from build123d import *

# Parameters (mm, degrees)
CROQUIS1_R              = 21
SALIENTE_EXTRUIR1_DEPTH = 5
CROQUIS2_R              = 12.5
CORTAR_EXTRUIR1_DEPTH   = 0.5
CROQUIS3_R              = 11
SALIENTE_EXTRUIR2_DEPTH = 2
CROQUIS4_R              = 2.5
CORTAR_EXTRUIR2_DEPTH   = 7.5
REDONDEO1_R             = 0.5
REDONDEO2_R             = 0.5


with BuildPart() as part:
    # Croquis1 → Saliente-Extruir1 (new body)
    with BuildSketch(Plane.XY):
        Circle(CROQUIS1_R)
    extrude(amount=SALIENTE_EXTRUIR1_DEPTH)

    # Croquis2 → Cortar-Extruir1 (cut)
    with BuildSketch(Plane.XY.offset(5)):
        Circle(CROQUIS2_R)
    extrude(amount=-CORTAR_EXTRUIR1_DEPTH, mode=Mode.SUBTRACT)

    # Croquis3 → Saliente-Extruir2 (add)
    with BuildSketch(Plane.XY.offset(4.5)):
        Circle(CROQUIS3_R)
    extrude(amount=SALIENTE_EXTRUIR2_DEPTH)

    # Croquis4 → Cortar-Extruir2 (cut, through all)
    with BuildSketch(Plane.XY.offset(6.5)):
        Circle(CROQUIS4_R)
    extrude(amount=-CORTAR_EXTRUIR2_DEPTH, mode=Mode.SUBTRACT)

    # Redondeo1
    redondeo1_edges = [part.edges().sort_by_distance(p)[0] for p in [
        (-21, 0, 5),
    ]]
    fillet(redondeo1_edges, radius=REDONDEO1_R)

    # Redondeo2
    redondeo2_edges = [part.edges().sort_by_distance(p)[0] for p in [
        (-11, 0, 6.5),
    ]]
    fillet(redondeo2_edges, radius=REDONDEO2_R)


solid = part.part
Input: part model. Units: mm. Frame: model coordinates. A direction names the side the tool comes from. Coordinates: 2 decimals unless noted, no trailing zeros. Loops run counter-clockwise (first coordinate to the right, second up) from the corner with the lowest first, then second, coordinate; pieces in that order, holes last.
(1) Pull-direction query (X, two-part tool) for faces 3 (the face through (20.03, 6.31, 2.22)), 4 (the face through (9, 9, 5)), 5 (the face through (5, -10, 4.5)); classes: released by +X, released by -X, zero draft, split by the parting line, or undercut.
(2) Section C-C on z = 2. Return the cut outline in (x, y), then the cut area to 3 significant figures.
(3) Section A-A on x = 0. Return the cut outline in (y, z).
(4) First-contact query: pin 1 Ø12.5 at (x, y) = (8.5, -7.5) entering from +Z; pin 2 Ø8 at (x, y) = (-7, -13.5) entering from +Z; pin 3 Ø1.5 at (y, z) = (15, 3) entering from -X. Flat tips, straight axial feed; report the tip coordinate or a pass-through.
(5) Set-up query: faces 1 (the face through (2, -2, 6.5)), 2 (the face through (11.923, 3.755, 4.754)). Return all of +Z, -Z, +X, -X, +Y, -Y with unobstructed straight access to the full face (end or side cutting, diameter ignored); none if empty.
(6) Material intervals for probe 1 along Y at (x, z) = (0, 4.7); probe 2 along Y at (x, z) = (0, 4.9); probe 3 along X at (y, z) = (-1, 4.75), sorted ascending.
Data:
1. face 3: split by the parting line
1. face 4: zero draft
1. face 5: undercut
2. outline: circle Ø42 at (0, 0); hole circle Ø5 at (0, 0)
2. area: 1,370 mm2
3. outline: (-21, 0) - (-2.5, 0) - (-2.5, 6.5) - (-10.5, 6.5) arc R0.5 ccw to (-11, 6) - (-11, 4.5) - (-12.5, 4.5) - (-12.5, 5) - (-20.5, 5) arc R0.5 ccw to (-21, 4.5) - close; (2.5, 0) - (21, 0) - (21, 4.5) arc R0.5 ccw to (20.5, 5) - (12.5, 5) - (12.5, 4.5) - (11, 4.5) - (11, 6) arc R0.5 ccw to (10.5, 6.5) - (2.5, 6.5) - close
4. pin 1: stops at z = 6.5
4. pin 2: stops at z = 5
4. pin 3: stops at x = -15.43
5. face 1: +Z, +X, -X, +Y, -Y
5. face 2: +Z
6. probe 1: y = -20.96 to -12.5, -11 to -2.5, 2.5 to 11, 12.5 to 20.96
6. probe 2: y = -20.8 to -12.5, -11 to -2.5, 2.5 to 11, 12.5 to 20.8
6. probe 3: x = -20.91 to -12.46, -10.95 to -2.29, 2.29 to 10.95, 12.46 to 20.91
